Work out the finished part from the listing and answer in its coordinate system (mm). A direction names the side the tool comes from. Coordinates: 2 decimals unless noted, no trailing zeros. Write each loop counter-clockwise with the first axis right and the second up, starting at its lowest first coordinate (ties: lowest second). Pieces come first, ordered by that corner, then holes. Notation, with made-up numbers: (57, 53.5) - (112, 53.5) arc R35 cw to (112, 86.5) - close; hole circle Ø10 at (52.25, 34.25). An arc over 180 degrees is marked (long way). Use CSV: the item, a comma, the result in double quotes. Start each with the question number.
from build123d import *

# Parameters (mm, degrees)
F0_W     = 77.532463
F0_H     = 27.835902
F1_DEPTH = 17.78
F2_W     = 78.115414
F2_H     = 37.45459
F3_DEPTH = 18.034
F4_W     = 15.156722
F4_H     = 15.593934
F4_W_2   = 17.48852
F5_DEPTH = 15.494
F6_SIZE  = 15.24


with BuildPart() as f1:
    # F0 (on Front) → F1 (new body)
    with BuildSketch(Plane.XZ):
        with Locations((3.497705, 13.917951)):
            Rectangle(F0_W, F0_H)
        Polygon((-20.694755, 45.324426), (-35.268527, 27.835902), (42.263936, 27.835902), (26.232786, 45.324426), align=None)
    extrude(amount=F1_DEPTH)

    # F2 (on Top) → F3 (join)
    with BuildSketch(Plane.XY):
        with Locations((3.497703, -18.727295)):
            Rectangle(F2_W, F2_H)
        Polygon((25.35836, -55.817544), (42.55541, -37.45459), (-35.560004, -37.45459), (-18.362952, -55.817544), align=None)
    extrude(amount=-F3_DEPTH)

    # F4 (on face) → F5 (join)
    with BuildSketch(Plane.XZ.offset(17.78)):
        with Locations((-18.945902, 7.796967)):
            Rectangle(F4_W, F4_H)
        with Locations((24.192458, 7.796967)):
            Rectangle(F4_W_2, F4_H)
    extrude(amount=F5_DEPTH)

    # F6
    f6_edges = [f1.edges().sort_by_distance(p)[0] for p in [
        (-18.945902, -33.274, 15.593934),
        (24.192458, -33.274, 15.593934),
    ]]
    chamfer(f6_edges, length=F6_SIZE)


solid = f1.part
Item 1: A cutting plane is placed at C-C (z = 8). Determine the outline of the cut face in (x, y).
Item 2: Straight lines are drawn through the part: probe 1 along Z at (x, y) = (-25, -39); probe 2 along Y at (x, z) = (-13.5, 37); probe 3 along Y at (x, z) = (28.5, 7.5). For each, find the intervals that lie inside material, in ascending order. Write a range as [from, to].
Item 3: A cutting plane is placed at B-B (y = -15). Determine the outline of the cut face in (x, z), then the cut area to 3 significant figures.
Item 4: Which of the six approach directions +Z, -Z, +X, -X, +Y, -Y give full straight-line access (tool end or side, diameter ignored) to faces 5 (the face through (-26.524, -24, 6)), 6 (the face through (-19.05, -25.55, 8.08)), 7 (the face through (42.264, -9, 14)), 8 (the face through (15.448, -24, 6)), 9 (the face through (-35.269, -9, 14))?
Item 5: Each of these flat-tipped pins is pushed along its axis until it touches: pin 1 (12 mm diameter, centred on y = -26.5, z = 7.5, fed in from +X); pin 2 (1 mm diameter, centred on x = 21.5, z = 6, fed in from -Y); pin 3 (10 mm diameter, centred on y = -6, z = 38, fed in from +X). Where does it stop, or does it pass through?
Item 6: Determine the mould class of faces 1 (the face through (-11.368, -24, 6)), 2 (the face through (3, -28, -18.034)), 3 (the face through (32.937, -24, 6)), 4 (the face through (3, -40, 0)) for opening direction X: +X half, -X half, draft (parallel to the pull), parting line (faces both ways), or undercut.
Item 7: A cutting plane is placed at D-D (x = 3). Determine the outline of the cut face in (y, z), then the cut area to 3 significant figures.
Item 8: A cutting plane is placed at A-A (x = -14). Determine the outline of the cut face in (y, z).
Calculated:
1,outline,"(-35.27, -17.78) - (-26.52, -17.78) - (-26.52, -25.63) - (-11.37, -25.63) - (-11.37, -17.78) - (15.45, -17.78) - (15.45, -25.63) - (32.94, -25.63) - (32.94, -17.78) - (42.26, -17.78) - (42.26, 0) - (-35.27, 0) - close"
2,probe 1,"z = [-18.03, 0]"
2,probe 2,"y = [-17.78, 0]"
2,probe 3,"y = [-26.13, 0]"
3,outline,"(-35.56, -18.03) - (42.56, -18.03) - (42.56, 0) - (42.26, 0) - (42.26, 27.84) - (26.23, 45.32) - (-20.69, 45.32) - (-35.27, 27.84) - (-35.27, 0) - (-35.56, 0) - close"
3,area,"4,660 mm²"
4,face 5,"+Z, -X, -Y"
4,face 6,"+Z, +X, -X, -Y"
4,face 7,"+Z, +X, +Y, -Y"
4,face 8,"+Z, -Y"
4,face 9,"+Z, -X, +Y, -Y"
5,pin 1,"stops at x = 32.94"
5,pin 2,"stops at y = -28.13"
5,pin 3,"stops at x = 37.53"
6,face 1,"undercut"
6,face 2,"draft"
6,face 3,"+X half"
6,face 4,"undercut"
7,outline,"(-55.82, -18.03) - (0, -18.03) - (0, 45.32) - (-17.78, 45.32) - (-17.78, 0) - (-55.82, 0) - close"
7,area,"1,810 mm²"
8,outline,"(-55.82, -18.03) - (0, -18.03) - (0, 45.32) - (-17.78, 45.32) - (-17.78, 15.59) - (-18.03, 15.59) - (-33.27, 0.35) - (-33.27, 0) - (-55.82, 0) - close"
